```python
from build123d import *

# Parameters (mm, degrees)
F1_DEPTH = 2
F2_SIZE  = 0.4


# Not quite as in the source:
# - a feature names something its author has since deleted; it is built from what else it names


with BuildPart() as f1:
    # F0 (on Top) → F1 (new body)
    with BuildSketch(Plane.XY):
        with BuildLine():
            Line((-8.3299736083, -24.3851770833), (-12.3299736083, -24.3851770833))
            Line((-12.3299736083, -24.3851770833), (-12.3299736083, -35.3851770833))
            Line((-12.3299736083, -35.3851770833), (-8.3299736083, -35.3851770833))
            ThreePointArc((-8.3299736083, -35.3851770833), (-2.8299736083, -29.8851770833), (-8.3299736083, -24.3851770833))
        make_face()
        with BuildLine():
            Line((-10.3299736083, -33.3851770833), (-10.3299736083, -26.3851770833))
            Line((-10.3299736083, -26.3851770833), (-8.3299736083, -26.3851770833))
            ThreePointArc((-8.3299736083, -26.3851770833), (-4.8299736083, -29.8851770833), (-8.3299736083, -33.3851770833))
            Line((-8.3299736083, -33.3851770833), (-10.3299736083, -33.3851770833))
        make_face(mode=Mode.SUBTRACT)
    extrude(amount=F1_DEPTH)

    # F2
    f2_edges = [f1.edges().sort_by_distance(p)[0] for p in [
        (-9.329974, -33.385177, 2),
        (-10.329974, -29.885177, 2),
        (-9.329974, -26.385177, 2),
        (-10.329974, -35.385177, 2),
        (-12.329974, -29.885177, 2),
        (-12.329974, -35.385177, 1),
        (-10.329974, -24.385177, 2),
        (-12.329974, -24.385177, 1),
        (-12.329974, -29.885177, 0),
        (-10.329974, -29.885177, 0),
        (-9.329974, -26.385177, 0),
        (-10.329974, -24.385177, 0),
        (-9.329974, -33.385177, 0),
        (-10.329974, -35.385177, 0),
        (-2.829974, -29.885177, 0),
        (-2.829974, -29.885177, 2),
        (-4.829974, -29.885177, 0),
        (-4.829974, -29.885177, 2),
    ]]
    chamfer(f2_edges, length=F2_SIZE)


solid = f1.part
```
The model under review builds one solid part; all positions refer to its coordinate system, in mm. A direction names the side the tool comes from. Give positions to 0.01 mm unless a question says otherwise; leave off trailing zeros. Write each loop counter-clockwise with the first axis right and the second up, starting at its lowest first coordinate (ties: lowest second). Pieces come first, ordered by that corner, then holes. Notation, with made-up numbers: (13, 9) - (30, 9) arc R34 cw to (30, 39) - close; hole circle Ø9 at (1, 21.5). An arc over 180 degrees is marked (long way). Answer in a Markdown table with one row per item. Add a question column.
1. We need section B-B on x = -10. Write out the cut boundary in (y, z).
2. We need section A-A on z = 1.1. Write out the cut boundary in (x, y), then the cut area to 3 significant figures.
3. Insertion check: P1, Ø1, axis at x = -4.5, z = 1.5, coming from the +Y side. The pin has a flat end and moves straight along its axis. Give the tip position at first contact, or say it passes through.
4. Draft analysis for pull direction Y (two halves, no side actions). For faces 1 (the flat face through (-10.33, -30, 1)), 2 (the flat face through (-10, -35.385, 1)), 3 (the conical face through (-3.12, -30, 0.11)), 4 (the flat face through (-12.33, -30, 1)), state which applies: +Y half, -Y half, draft (parallel to the pull), parting line (faces both ways), or undercut.
5. We need section C-C on z = 0.15. Write out the cut boundary in (x, y).
6. Tool access review of faces 5 (the conical face through (-4.72, -29.81, 0.29)), 6 (the flat face through (-9, -26.385, 1)), 7 (the conical face through (-4.72, -29.81, 1.71)): name each direction out of +Z, -Z, +X, -X, +Y, -Y from which nothing blocks a thin tool from reaching the whole face with its end or side.
7. Wall thickness on line 1 along Y through (x, z) = (-8.25, 0.7); line 2 along X through (y, z) = (-31.75, 1.5); line 3 along X through (y, z) = (-26.75, 0.6): over which ranges is each line inside the solid? List them lowest first. Write a range as [from, to].
Ans:
| question | item | result |
|---|---|---|
| 1 | outline | (-35.39, 0.4) - (-34.99, 0) - (-33.79, 0) - (-33.39, 0.4) - (-33.39, 1.6) - (-33.79, 2) - (-34.99, 2) - (-35.39, 1.6) - close; (-26.39, 0.4) - (-25.99, 0) - (-24.79, 0) - (-24.39, 0.4) - (-24.39, 1.6) - (-24.79, 2) - (-25.99, 2) - (-26.39, 1.6) - close |
| 2 | outline | (-12.33, -34.99) - (-11.93, -35.39) - (-8.33, -35.39) arc R5.5 ccw to (-8.33, -24.39) - (-11.93, -24.39) - (-12.33, -24.79) - close; hole (-10.33, -33.39) - (-8.33, -33.39) arc R3.5 ccw to (-8.33, -26.39) - (-10.33, -26.39) - close |
| 2 | area | 58.1 mm^2 |
| 3 | P1 | stops at y = -25.51 |
| 4 | face 1 | undercut |
| 4 | face 2 | -Y half |
| 4 | face 3 | parting line |
| 4 | face 4 | draft |
| 5 | outline | (-12.08, -34.99) - (-11.93, -35.14) - (-8.33, -35.14) arc R5.25 ccw to (-8.33, -24.64) - (-11.93, -24.64) - (-12.08, -24.79) - close; hole (-10.58, -33.64) - (-8.33, -33.64) arc R3.75 ccw to (-8.33, -26.14) - (-10.58, -26.14) - close |
| 6 | face 5 | -Z |
| 6 | face 6 | +Z, -Z |
| 6 | face 7 | +Z |
| 7 | line 1 | y = [-35.38, -33.38], [-26.39, -24.39] |
| 7 | line 2 | x = [-12.33, -10.33], [-5.37, -3.16] |
| 7 | line 3 | x = [-12.33, -10.33], [-6.77, -3.81] |
